Build history of the part. All positions in model axes, mm. A direction names the side the tool comes from. Round coordinates to 2 decimals unless told otherwise and drop trailing zeros. Write each loop counter-clockwise with the first axis right and the second up, starting at its lowest first coordinate (ties: lowest second). Pieces come first, ordered by that corner, then holes. Notation, with made-up numbers: (84, 8.25) - (124, 8.25) arc R15 cw to (124, 30.25) - close; hole circle Ø9 at (14.5, 64). An arc over 180 degrees is marked (long way). Write each question's results on one line, items separated by ' | '.
from build123d import *

# Parameters (mm, degrees)
F0_W     = 3.175
F0_H     = 25.4
F0_H_2   = 11.43
F2_DEPTH = 10.16
F3_R     = 5.08


with BuildPart() as f1:
    # F0 (on Front) → F1 (revolve)
    with BuildSketch(Plane.XZ):
        Polygon((-31.75, 0), (0, 0), (0, 3.175), (-28.575, 3.175), (-28.575, 128.27), (-31.75, 128.27), align=None)
        with Locations((-30.1625, 152.4)):
            Rectangle(F0_W, F0_H)
        with Locations((-30.1625, 133.985)):
            Rectangle(F0_W, F0_H_2)
    revolve(axis=Axis((0, 0, 1.5875), (0, 0, 1)))

    # F0 (on Front) → F2 (join, symmetric)
    with BuildSketch(Plane.XZ):
        Polygon((-38.349897, 128.27), (-31.75, 128.27), (-31.75, 139.7), (-44.45, 139.7), (-69.215, 86.591286), (-57.785, 86.591286), align=None)
        with Locations((-30.1625, 133.985)):
            Rectangle(F0_W, F0_H_2)
    extrude(amount=F2_DEPTH, both=True)

    # F3
    f3_edges = [f1.edges().sort_by_distance(p)[0] for p in [
        (-56.8325, 10.16, 113.145643),
        (-56.8325, -10.16, 113.145643),
        (-37.265253, -10.16, 139.7),
        (-37.265253, 10.16, 139.7),
        (-44.45, 0, 139.7),
        (-48.067448, -10.16, 107.430643),
        (-48.067448, 10.16, 107.430643),
        (-63.5, -10.16, 86.591286),
        (-63.5, 10.16, 86.591286),
        (-57.785, 0, 86.591286),
        (-69.215, 0, 86.591286),
        (-34.215202, 10.16, 128.27),
        (-34.215202, -10.16, 128.27),
    ]]
    fillet(f3_edges, radius=F3_R)


solid = f1.part
(1) Slice it at B-B, the plane y = 0. Write the cut outline in (x, z) (3 decimals), and give its area (3 significant figures).
Worked answers:
outline: (-65.845, 93.818) arc R5.08 ccw to (-61.241, 86.591) - (-61.021, 86.591) arc R5.08 ccw to (-56.417, 89.524) - (-38.35, 128.27) - (-31.75, 128.27) - (-31.75, 0) - (31.75, 0) - (31.75, 165.1) - (28.575, 165.1) - (28.575, 3.175) - (-28.575, 3.175) - (-28.575, 165.1) - (-31.75, 165.1) - (-31.75, 139.7) - (-41.214, 139.7) arc R5.08 ccw to (-45.818, 136.767) - close | area: 1,860 mm2
(2) Slice it at D-D, the plane z = 115.5. State how many separate pieces and enclosed holes the cut face has, and give its area (3 significant figures).
Worked answers:
separate pieces: 2 | enclosed holes: 1 | area: 810 mm2
(3) Tool access for faces 1 (the flat face through (-41, -10.16, 134)), 2 (the cylindrical face through (-35.753, 8.632, 129.719)), 3 (the flat face through (0, 0, 3.175)): list every direction of +Z, -Z, +X, -X, +Y, -Y with a clear straight run to the whole face (end or side of a thin tool).
Worked answers:
face 1: +Z, -Z, -X, -Y | face 2: -Z, +Y | face 3: +Z
(4) Two-plate mould, pull along X, no slides. Class faces 4 (the flat face through (-47.51, -0.07, 108.63)), 5 (the cylindrical face through (-35.725, -8.632, 138.251)), 6 (the cylindrical face through (-43.909, -0.071, 138.926)): released by +X, released by -X, zero draft, split by the parting line, or undercut.
Worked answers:
face 4: undercut | face 5: zero draft | face 6: released by -X
(5) Slice it at A-A, the plane x = 0. Write the cut outline in (y, z) (3 decimals), and give its area (3 significant figures).
Worked answers:
outline: (-31.75, 0) - (31.75, 0) - (31.75, 165.1) - (28.575, 165.1) - (28.575, 3.175) - (-28.575, 3.175) - (-28.575, 165.1) - (-31.75, 165.1) - close | area: 1,230 mm2
(6) Drill centre lines: probe 1 along Y at (x, z) = (0, 59.5) (3 decimals); probe 2 along X at (y, z) = (0, 112) (3 decimals). Where is each one in solid material? Low to high. Write a range as [from, to].
Worked answers:
probe 1: y = [-31.75, -28.575], [28.575, 31.75] | probe 2: x = [-57.367, -45.937], [-31.75, -28.575], [28.575, 31.75]
(7) Slice it at C-C, the plane z = 57.5. Write the cut outline in (x, y) (3 decimals).
Worked answers:
outline: circle Ø63.5 at (0, 0); hole circle Ø57.15 at (0, 0)
(8) Flat gauge pins, fed straight in: pin 1 Ø3 at (x, y) = (-38.5, 1.5) entering from +Z; pin 2 Ø17 at (x, y) = (-9.5, -4.5) entering from +Z (3 decimals); pin 3 Ø8 at (x, z) = (-18.5, 41) entering from -Y. Where does each tip first touch, or does it go through?
Worked answers:
pin 1: stops at z = 139.7 | pin 2: stops at z = 3.175 | pin 3: stops at y = -28.25
